The model under review builds one solid part; all positions refer to its coordinate system, in mm. A direction names the side the tool comes from. Coordinates: 2 decimals unless noted, no trailing zeros. Write each loop counter-clockwise with the first axis right and the second up, starting at its lowest first coordinate (ties: lowest second). Pieces come first, ordered by that corner, then holes. Notation, with made-up numbers: (83, 41) - (110, 41) arc R24 ccw to (110, 70) - close; hole circle Ø2 at (-17, 80). An arc over 180 degrees is marked (long way). Put each result on its own line as item: value. Start each with the question number.
Item 1: Consider section C-C on z = 0.8. Give the boundary of the cut face in (x, y).
Item 2: To check wall thickness, follow L1, parallel to X at y = 2.25, z = 0.9; L2, parallel to X at y = 4, z = 2.9; L3, parallel to Y at x = -11.25, z = 3.65. State the ranges of each line that lie inside material, in increasing order. Write a range as [from, to].
Item 3: For pin 1 (1.6 mm diameter, centred on x = -3.5, z = 1, fed in from +Y); pin 2 (1.5 mm diameter, centred on x = -1, y = 4.5, fed in from +Z), all flat-tipped, find the tip position at first contact; note any pin that passes through.
Item 4: Consider section A-A on y = 6.5. Give the boundary of the cut face in (x, z), then the cut area to 3 significant figures.
Item 5: Consider section D-D on y = -0.5. Give the boundary of the cut face in (x, z).
Item 6: Consider section B-B on z = 3.2. State how many separate pieces and enclosed holes the cut face has, then the cut area to 3 significant figures.
Item 7: Machinability: for faces 1 (the face through (0.5, 1, 1)), 2 (the face through (-3.324, -2.43, 3.359)), 3 (the face through (-5, -2, 2.7)), 4 (the face through (-5.266, -2.43, 3.359)), which of the approach directions +Z, -Z, +X, -X, +Y, -Y give a long, thin tool a straight path to every point of the face, cutting with its end or side? Answer none if there is none.
Item 8: Mouldability with a two-part tool opening along X and no side actions: class faces 5 (the face through (14.5, 0, 2)), 6 (the face through (-3.77, -2.57, 3.36)), 7 (the face through (0, -7.5, 2)) as pulls with the +X half, pulls with the -X half, needs draft (parallel to the pull), parting line crosses it, or undercut.
```python
from build123d import *

# Parameters (mm, degrees)
PAD_DEPTH       = 4
SKETCH001_W     = 12
SKETCH001_H     = 2.5
POCKET_DEPTH    = 2
POCKET001_DEPTH = 1.3


with BuildPart() as part:
    # Sketch → Pad (new body)
    with BuildSketch(Plane.XY):
        Polygon((-14.5, 7.5), (-11.5, 7.5), (-11.5, 2.5), (11.5, 2.5), (11.5, 7.5), (14.5, 7.5), (14.5, -7.5), (-14.5, -7.5), align=None)
    extrude(amount=PAD_DEPTH)

    # Sketch001 (on Face9 of Pad) → Pocket (cut)
    with BuildSketch(Plane(origin=(0, 0, 0), x_dir=(1, 0, 0), z_dir=(0, 0, -1))):
        with Locations((-5.5, -1.25)):
            Rectangle(SKETCH001_W, SKETCH001_H)
    extrude(amount=-POCKET_DEPTH, mode=Mode.SUBTRACT)

    # Sketch002 (on Face5 of Pocket) → Pocket001 (cut)
    with BuildSketch(Plane.XY.offset(4)):
        Polygon((-5.050715, 2.5), (-5.487324, -7.5), (-3.985895, -7.5), (-3.549285, 2.5), align=None)
        Polygon((-3.539285, 2.5), (-3.102676, -7.5), (-1.601247, -7.5), (-2.037856, 2.5), align=None)
    extrude(amount=-POCKET001_DEPTH, mode=Mode.SUBTRACT)


solid = part.part
```
Report:
1. outline: (-14.5, -7.5) - (14.5, -7.5) - (14.5, 7.5) - (11.5, 7.5) - (11.5, 2.5) - (0.5, 2.5) - (0.5, 0) - (-11.5, 0) - (-11.5, 7.5) - (-14.5, 7.5) - close
2. L1: [-14.5, -11.5], [0.5, 14.5]
2. L2: [-14.5, -11.5], [11.5, 14.5]
2. L3: [-7.5, 2.5]
3. pin 1: y = 0
3. pin 2: through
4. outline: (-14.5, 0) - (-11.5, 0) - (-11.5, 4) - (-14.5, 4) - close; (11.5, 0) - (14.5, 0) - (14.5, 4) - (11.5, 4) - close
4. area: 24.0 mm²
5. outline: (-14.5, 0) - (14.5, 0) - (14.5, 4) - (-1.91, 4) - (-1.91, 2.7) - (-3.41, 2.7) - (-3.41, 4) - (-3.68, 4) - (-3.68, 2.7) - (-5.18, 2.7) - (-5.18, 4) - (-14.5, 4) - close
6. separate pieces: 3
6. enclosed holes: 0
6. area: 290 mm²
7. face 1: -Z, +Y
7. face 2: +Z, +Y
7. face 3: +Z
7. face 4: +Z, -Y
8. face 5: pulls with the +X half
8. face 6: undercut
8. face 7: needs draft
